For this review, use the dimensioned drawing (mm, ordinates from the lowest corner) and the shaded views. Coordinates: 2 decimals unless noted, no trailing zeros. Write each loop counter-clockwise with the first axis right and the second up, starting at its lowest first coordinate (ties: lowest second). Pieces come first, ordered by that corner, then holes. Notation, with made-up numbers: (4, -25) - (18, -25) arc R25 cw to (18, -4) - close; hole circle Ø6 at (27.5, 46.25). An arc over 180 degrees is marked (long way). Answer as a JSON object with one key per item and string values.
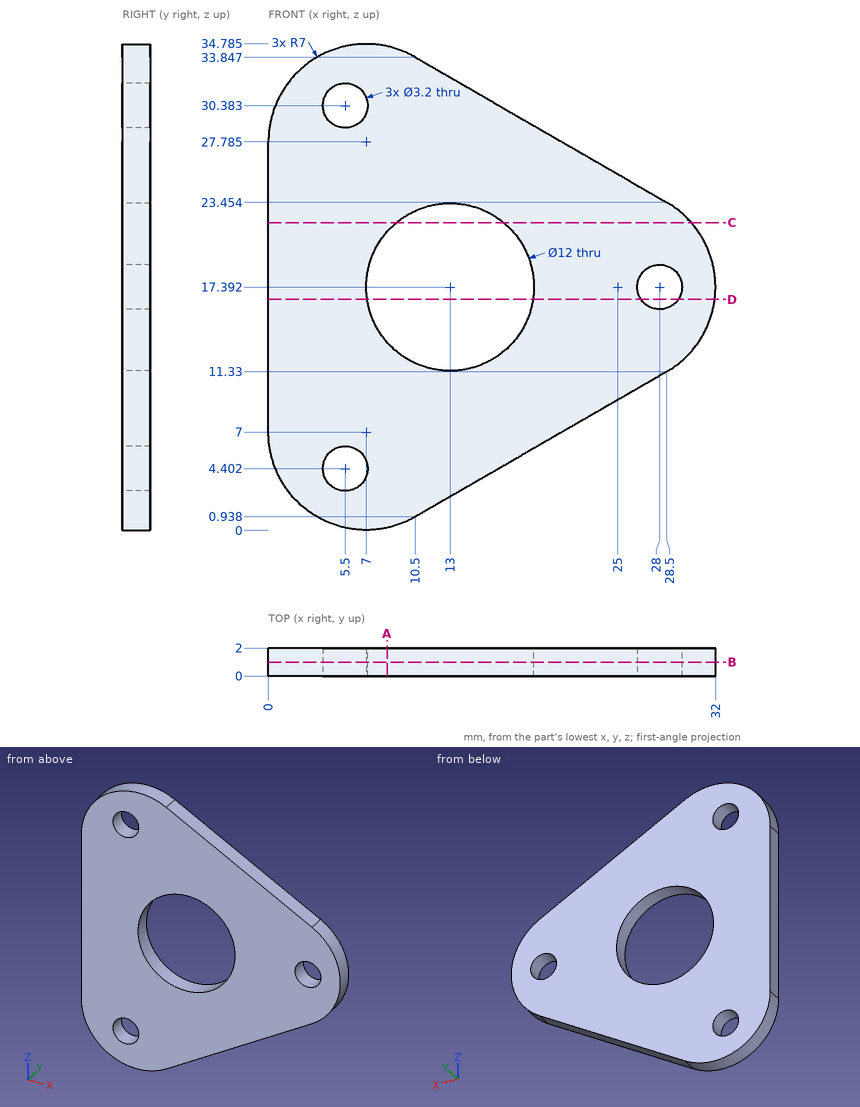
(1) Take a section at D-D, the plane z = 16.5. Write out the cut boundary in (x, y).
Solved:
{"outline": "(0, 0) - (7.07, 0) - (7.07, 2) - (0, 2) - close; (18.93, 0) - (26.67, 0) - (26.67, 2) - (18.93, 2) - close; (29.33, 0) - (31.94, 0) - (31.94, 2) - (29.33, 2) - close"}
(2) Take a section at A-A, the plane x = 8.5. Write out the cut boundary in (y, z).
Solved:
{"outline": "(0, 0.16) - (2, 0.16) - (2, 13.42) - (0, 13.42) - close; (0, 21.36) - (2, 21.36) - (2, 34.62) - (0, 34.62) - close"}
(3) Take a section at B-B, the plane y = 1. Write out the cut boundary in (x, z) (1 decimal).
Solved:
{"outline": "(0, 7) arc R7 ccw to (10.5, 0.9) - (28.5, 11.3) arc R7 ccw to (28.5, 23.5) - (10.5, 33.8) arc R7 ccw to (0, 27.8) - close; hole circle Ø3.2 at (5.5, 4.4); hole circle Ø3.2 at (5.5, 30.4); hole circle Ø12 at (13, 17.4); hole circle Ø3.2 at (28, 17.4)"}
(4) For pin 1 (1 mm diameter, centred on y = 0.5, z = 11.5, fed in from +X) (1 decimal), flat-tipped, find the tip position at first contact; note if it passes through.
Solved:
{"pin 1": "stops at x = 29.5"}
(5) Take a section at C-C, the plane z = 22. Write out the cut boundary in (x, y).
Solved:
{"outline": "(0, 0) - (9.16, 0) - (9.16, 2) - (0, 2) - close; (16.84, 0) - (30.27, 0) - (30.27, 2) - (16.84, 2) - close"}
(6) To check wall thickness, follow line 1 (X direction, y = 1.4, z = 17); line 2 (Z direction, x = 5, y = 0.55); line 3 (Z direction, x = 6, y = 1.7). State the ranges of each line that lie inside material, in increasing order. Write a range as from..to.
Solved:
{"line 1": "x = 0..7.01, 18.99..26.45, 29.55..31.99", "line 2": "z = 0.29..2.88, 5.92..28.86, 31.9..34.49", "line 3": "z = 0.07..2.88, 5.92..28.86, 31.9..34.71"}
